Build history of the part. All positions in model axes, mm. Face numbers are marked on the shaded views. A direction names the side the tool comes from. Round coordinates to 2 decimals unless told otherwise and drop trailing zeros. Write each loop counter-clockwise with the first axis right and the second up, starting at its lowest first coordinate (ties: lowest second). Pieces come first, ordered by that corner, then holes. Notation, with made-up numbers: M 88,51 L 145,51 A25 cw 145,69 Z; hole C 36.5,60.5 d11. An arc over 180 degrees is marked long. Write item = value, one per line.
Autodesk Inventor part; units mm, degrees
ref_plane "YZ Plane" through (0, 0, 0) normal (1, 0, 0) x (0, 1, 0)
ref_plane "XZ Plane" through (0, 0, 0) normal (0, 1, 0) x (-1, 0, 0)
ref_plane "XY Plane" through (0, 0, 0) normal (0, 0, 1) x (1, 0, 0)
sketch "スケッチ1" plane through (0, 0, 0) normal (0, 1, 0) x (-1, 0, 0)
  line L0 (8.5, 15.5) -> (-8.5, 15.5)
  line L1 (-8.5, 15.5) -> (-8.5, -15.5)
  line L2 (-8.5, -15.5) -> (8.5, -15.5)
  line L3 (8.5, -15.5) -> (8.5, 15.5)
  circle A0 centre (0, 9.2) radius 6.3
  circle A1 centre (0, -9.2) radius 6.3
  circle A2 centre (6.75, -13.5) radius 1.1
  line L4 (6.75, -13.5) -> (-6.75, -13.5) construction
  line L5 (-6.75, -13.5) -> (-6.75, 13.5) construction
  line L6 (-6.75, 13.5) -> (6.75, 13.5) construction
  line L7 (6.75, 13.5) -> (6.75, -13.5) construction
  circle A3 centre (-6.75, -13.5) radius 1.1
  circle A4 centre (6.75, 13.5) radius 1.1
  circle A5 centre (-6.75, 13.5) radius 1.1
  point P0 (0, 0)
  point P1 (0, 15.5)
  point P2 (8.5, 0)
  point P3 (6.75, 0)
  point P4 (0, 13.5)
  dimension "d0" = 17
  dimension "d1" = 31
  dimension "d2" = 12.6
  dimension "d10" = 2.2
  dimension "d11" = 27
  dimension "d12" = 13.5
  dimension "d13" = 2.2
  dimension "d14" = 2.2
  dimension "d15" = 2.2
  dimension "d16" = 9.2
extrude "押し出し1" add sketch "スケッチ1" along normal blind 1.6 contours A0 | A1 | L3 L2 L1 L0
extrude "押し出し2" add sketch "スケッチ1" against normal blind 9 contours A0 | A1
sketch "スケッチ2" plane through (0, 1.6, 0) normal (0, 1, 0) x (1, 0, 0)
  line L0 (8.5, 15.5) -> (-8.5, 15.5)
  line L1 (-8.5, 15.5) -> (-8.5, -15.5)
  line L2 (-8.5, -15.5) -> (8.5, -15.5)
  line L3 (8.5, -15.5) -> (8.5, 15.5)
  line L4 (-5.5, -12.5) -> (-5.5, 12.5)
  line L5 (-5.5, 12.5) -> (5.5, 12.5)
  line L6 (5.5, 12.5) -> (5.5, -12.5)
  line L7 (5.5, -12.5) -> (-5.5, -12.5)
  point P0 (0, 0)
  dimension "d7" = 3
extrude "押し出し3" add sketch "スケッチ2" along normal blind 1.6 contours L4 L5 L6 L7
properties part number "UltrasonicSensor"
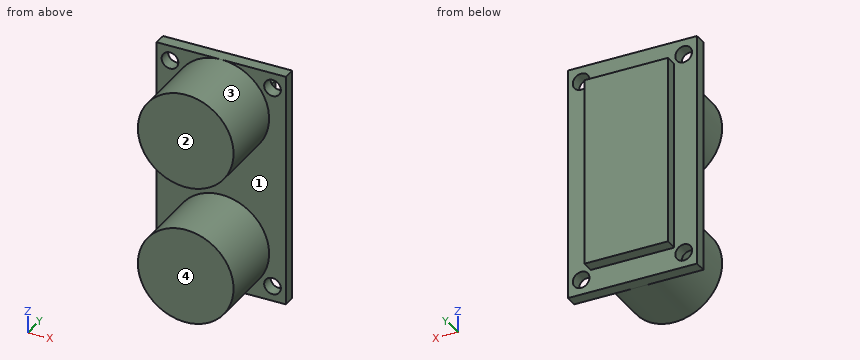
1. Band-saw the part on A-A (x = 6.75). List the corners of the cut face in (y, z).
Responses:
outline = M 0,-15.5 L 1.6,-15.5 L 1.6,-14.6 L 0,-14.6 Z; M 0,-12.4 L 1.6,-12.4 L 1.6,12.4 L 0,12.4 Z; M 0,14.6 L 1.6,14.6 L 1.6,15.5 L 0,15.5 Z
2. Probe probe 1 along Z at (x, y) = (6.75, 1); probe 2 along Z at (x, y) = (-1.75, -3.5); probe 3 along Z at (x, y) = (1, -3.75). List the from-to ranges inside material, lowest first.
Responses:
probe_1 = -15.5 to -14.6, -12.4 to 12.4, 14.6 to 15.5
probe_2 = -15.25 to -3.15, 3.15 to 15.25
probe_3 = -15.42 to -2.98, 2.98 to 15.42
3. Band-saw the part on D-D (z = 1). List the corners of the cut face in (x, y).
Responses:
outline = M -8.5,0 L 8.5,0 L 8.5,1.6 L 5.5,1.6 L 5.5,3.2 L -5.5,3.2 L -5.5,1.6 L -8.5,1.6 Z
4. Mould opens along Z. For the marked faces 3 and 4 say: pulls with the +Z half, pulls with the -Z half, needs draft (parallel to the pull), parting line crosses it, or undercut.
Responses:
face_3 = undercut
face_4 = needs draft
5. Flat gauge pins, fed straight in: pin 1 (3 mm diameter, centred on x = 6.75, z = 13.5, fed in from -Y); pin 2 (1 mm diameter, centred on x = 2.5, y = -1, fed in from -Z); pin 3 (3 mm diameter, centred on x = -6, z = 11.5, fed in from +Y); pin 4 (5 mm diameter, centred on y = -7.5, z = -10.5, fed in from -X). Where does each tip first touch, or does it go through?
Responses:
pin_1 = 0
pin_2 = -15.17
pin_3 = 3.2
pin_4 = -6.3
6. Band-saw the part on B-B (y = -7.25). List the corners of the cut face in (x, z).
Responses:
outline = C 0,-9.2 d12.6; C 0,9.2 d12.6
7. Tool access for the marked faces 1 and 2: list every direction of +Z, -Z, +X, -X, +Y, -Y with a clear straight run to the whole face (end or side of a thin tool).
Responses:
face_1 = -Y
face_2 = +Z, -Z, +X, -X, -Y
8. Band-saw the part on C-C (z = -13.5). List the corners of the cut face in (x, y), plus the area to 3 significant figures.
Responses:
outline = M -8.5,0 L -7.85,0 L -7.85,1.6 L -8.5,1.6 Z; M -5.65,0 L -4.6,0 L -4.6,-9 L 4.6,-9 L 4.6,0 L 5.65,0 L 5.65,1.6 L -5.65,1.6 Z; M 7.85,0 L 8.5,0 L 8.5,1.6 L 7.85,1.6 Z
area = 103 mm²
